```python
from build123d import *

# Parameters (mm, degrees)
F0_R         = 12.5
F1_DEPTH     = 12.5
F2_R         = 2.25
F3_DEPTH     = 25
F4_R         = 12.5
F5_DEPTH     = 7.5
F6_R         = 12.5
F7_DEPTH     = 7.5
F8_T4_DEPTH  = 24.3016555368
F8_S5_R      = 12.5
F8_T6_DEPTH  = 15
F8_T11_DEPTH = 24.3016555368
F8_S12_R     = 12.5
F8_T13_DEPTH = 14
F8_T17_DEPTH = 24.3016555368
F8_S18_R     = 12.5
F8_T19_DEPTH = 15
F8_T24_DEPTH = 24.3016555368
F8_S25_R     = 12.5
F8_T26_DEPTH = 15
F8_T30_DEPTH = 24.3016555368
F8_S31_R     = 12.5
F8_T32_DEPTH = 15
F8_T37_DEPTH = 24.3016555368
F8_S38_R     = 12.5
F8_T39_DEPTH = 15
F8_T44_DEPTH = 24.3016555368
F8_S45_R     = 12.5
F8_T46_DEPTH = 15
F9_T1_DEPTH  = 24.050587715
F9_T3_DEPTH  = 24.050587715
F9_T5_DEPTH  = 24.050587715
F9_T7_DEPTH  = 24.050587715
F9_T9_DEPTH  = 24.050587715
F9_T11_DEPTH = 24.050587715
F9_T13_DEPTH = 24.050587715
F10_R        = 2.5
F11_DEPTH    = 12


# Not quite as in the source:
# - a fillet or chamfer that OpenCascade refuses, or shapes differently, is made with other operations: its cross-section is extruded or revolved along the edge and cut away or added


with BuildPart() as f1:
    # F0 (on Top) → F1 (new body, symmetric)
    with BuildSketch(Plane.XY):
        Polygon((22.5, -5.1354781738), (22.5, 5.1354781738), (18.0435990556, 14.3892900865), (10.013442028, 20.7931266245), (0, 23.0786294236), (-10.013442028, 20.7931266245), (-18.0435990556, 14.3892900865), (-22.5, 5.1354781738), (-22.5, -5.1354781738), (-18.0435990556, -14.3892900865), (-10.013442028, -20.7931266245), (0, -23.0786294236), (10.013442028, -20.7931266245), (18.0435990556, -14.3892900865), align=None)
        Circle(F0_R, mode=Mode.SUBTRACT)
    extrude(amount=F1_DEPTH, both=True)

    # F2 (on face) → F3 (cut)
    with BuildSketch(Plane.XY.offset(12.5)):
        with Locations((9, 15.5884572681)):
            Circle(F2_R)
        with Locations((-18, 0)):
            Circle(F2_R)
        with Locations((9, -15.5884572681)):
            Circle(F2_R)
    extrude(amount=-F3_DEPTH, mode=Mode.SUBTRACT)

    # F4 (on face) → F5 (cut)
    with BuildSketch(Plane.XY.offset(12.5)):
        Polygon((14.9, -3.4008277684), (14.9, 3.4008277684), (11.9488722635, 9.5289076573), (6.6311238319, 13.7696705203), (0, 15.2831812628), (-6.6311238319, 13.7696705203), (-11.9488722635, 9.5289076573), (-14.9, 3.4008277684), (-14.9, -3.4008277684), (-11.9488722635, -9.5289076573), (-6.6311238319, -13.7696705203), (0, -15.2831812628), (6.6311238319, -13.7696705203), (11.9488722635, -9.5289076573), align=None)
        Circle(F4_R, mode=Mode.SUBTRACT)
    extrude(amount=-F5_DEPTH, mode=Mode.SUBTRACT)

    # F6 (on face) → F7 (join)
    with BuildSketch(Plane(origin=(0, 0, -12.5), x_dir=(1, 0, 0), z_dir=(0, 0, -1))):
        Polygon((14.35, -3.2752938575), (14.35, 3.2752938575), (11.5078065088, 9.1771694552), (6.3863508045, 13.2613940917), (0, 14.719036988), (-6.3863508045, 13.2613940917), (-11.5078065088, 9.1771694552), (-14.35, 3.2752938575), (-14.35, -3.2752938575), (-11.5078065088, -9.1771694552), (-6.3863508045, -13.2613940917), (0, -14.719036988), (6.3863508045, -13.2613940917), (11.5078065088, -9.1771694552), align=None)
        Circle(F6_R, mode=Mode.SUBTRACT)
    extrude(amount=F7_DEPTH)

    # F8: fillet of radius 3.5 on 7 edges, made by hand


with BuildPart() as f8_tool2:
    # F8_s3 → F8_t4 (new body)
    with BuildSketch(Plane(origin=(9.4998996874, 7.5759171977, 0), x_dir=(0, 0, 1), z_dir=(-0.7818314825, -0.6234898019, 0))):
        with BuildLine():
            ThreePointArc((5, 11.4), (6.0251262658, 13.8748737342), (8.5, 14.9))
            Line((8.5, 14.9), (5, 14.9))
            Line((5, 14.9), (5, 11.4))
        make_face()
    extrude(amount=F8_T4_DEPTH)

    # F8_s5 → F8_t6 (cut, symmetric)
    with BuildSketch(Plane.XY.offset(6.8)):
        Circle(F8_S5_R)
    extrude(amount=F8_T6_DEPTH, both=True, mode=Mode.SUBTRACT)

    split(bisect_by=Plane(origin=(-13.4244361317, 6.4648677129, 0), x_dir=(0, 0, 1), z_dir=(0.9009688679, -0.4338837391, 0)), keep=Keep.TOP)


with BuildPart() as f1_1:
    add(f1.part)

    # F8_t1: union F8_tool2
    add(f8_tool2.part)


with BuildPart() as f8_tool9:
    # F8_s10 → F8_t11 (new body)
    with BuildSketch(Plane.XZ.offset(-12.1508277684)):
        with BuildLine():
            ThreePointArc((-11.4, 5), (-13.8748737342, 6.0251262658), (-14.9, 8.5))
            Line((-14.9, 8.5), (-14.9, 5))
            Line((-14.9, 5), (-11.4, 5))
        make_face()
    extrude(amount=F8_T11_DEPTH)

    # F8_s12 → F8_t13 (cut, symmetric)
    with BuildSketch(Plane.XY.offset(6.8)):
        Circle(F8_S12_R)
    extrude(amount=F8_T13_DEPTH, both=True, mode=Mode.SUBTRACT)


with BuildPart() as f1_2:
    add(f1_1.part)

    # F8_t8: union F8_tool9
    add(f8_tool9.part)


with BuildPart() as f8_tool15:
    # F8_s16 → F8_t17 (new body)
    with BuildSketch(Plane(origin=(-9.4998996874, 7.5759171977, 0), x_dir=(0, 0, 1), z_dir=(0.7818314825, -0.6234898019, 0))):
        with BuildLine():
            ThreePointArc((5, 11.4), (6.0251262658, 13.8748737342), (8.5, 14.9))
            Line((8.5, 14.9), (5, 14.9))
            Line((5, 14.9), (5, 11.4))
        make_face()
    extrude(amount=F8_T17_DEPTH)

    # F8_s18 → F8_t19 (cut, symmetric)
    with BuildSketch(Plane.XY.offset(6.8)):
        Circle(F8_S18_R)
    extrude(amount=F8_T19_DEPTH, both=True, mode=Mode.SUBTRACT)

    split(bisect_by=Plane.YZ.offset(-14.9), keep=Keep.TOP)


with BuildPart() as f1_3:
    add(f1_2.part)

    # F8_t14: union F8_tool15
    add(f8_tool15.part)


with BuildPart() as f8_tool22:
    # F8_s23 → F8_t24 (new body)
    with BuildSketch(Plane(origin=(-11.8461811475, -2.7038135434, 0), x_dir=(0, 0, 1), z_dir=(0.9749279122, 0.222520934, 0))):
        with BuildLine():
            ThreePointArc((8.5, 14.9), (6.0251262658, 13.8748737342), (5, 11.4))
            Line((5, 11.4), (5, 14.9))
            Line((5, 14.9), (8.5, 14.9))
        make_face()
    extrude(amount=F8_T24_DEPTH)

    # F8_s25 → F8_t26 (cut, symmetric)
    with BuildSketch(Plane.XY.offset(6.8)):
        Circle(F8_S25_R)
    extrude(amount=F8_T26_DEPTH, both=True, mode=Mode.SUBTRACT)


with BuildPart() as f1_4:
    add(f1_3.part)

    # F8_t21: union F8_tool22
    add(f8_tool22.part)


with BuildPart() as f8_tool28:
    # F8_s29 → F8_t30 (new body)
    with BuildSketch(Plane(origin=(-5.2720465855, -10.9475175386, 0), x_dir=(0, 0, 1), z_dir=(0.4338837391, 0.9009688679, 0))):
        with BuildLine():
            ThreePointArc((5, 11.4), (6.0251262658, 13.8748737342), (8.5, 14.9))
            Line((8.5, 14.9), (5, 14.9))
            Line((5, 14.9), (5, 11.4))
        make_face()
    extrude(amount=F8_T30_DEPTH)

    # F8_s31 → F8_t32 (cut, symmetric)
    with BuildSketch(Plane.XY.offset(6.8)):
        Circle(F8_S31_R)
    extrude(amount=F8_T32_DEPTH, both=True, mode=Mode.SUBTRACT)

    split(bisect_by=Plane(origin=(9.2899980477, -11.6492890888, 0), x_dir=(0, 0, 1), z_dir=(-0.6234898019, 0.7818314825, 0)), keep=Keep.TOP)


with BuildPart() as f1_5:
    add(f1_4.part)

    # F8_t27: union F8_tool28
    add(f8_tool28.part)


with BuildPart() as f8_tool35:
    # F8_s36 → F8_t37 (new body)
    with BuildSketch(Plane(origin=(5.2720465855, -10.9475175386, 0), x_dir=(0, 0, 1), z_dir=(-0.4338837391, 0.9009688679, 0))):
        with BuildLine():
            ThreePointArc((5, 11.4), (6.0251262658, 13.8748737342), (8.5, 14.9))
            Line((8.5, 14.9), (5, 14.9))
            Line((5, 14.9), (5, 11.4))
        make_face()
    extrude(amount=F8_T37_DEPTH)

    # F8_s38 → F8_t39 (cut, symmetric)
    with BuildSketch(Plane.XY.offset(6.8)):
        Circle(F8_S38_R)
    extrude(amount=F8_T39_DEPTH, both=True, mode=Mode.SUBTRACT)

    split(bisect_by=Plane(origin=(9.2899980477, 11.6492890888, 0), x_dir=(0, 0, 1), z_dir=(-0.6234898019, -0.7818314825, 0)), keep=Keep.TOP)


with BuildPart() as f1_6:
    add(f1_5.part)

    # F8_t34: union F8_tool35
    add(f8_tool35.part)


with BuildPart() as f8_tool42:
    # F8_s43 → F8_t44 (new body)
    with BuildSketch(Plane(origin=(11.8461811475, -2.7038135434, 0), x_dir=(0, 0, 1), z_dir=(-0.9749279122, 0.222520934, 0))):
        with BuildLine():
            ThreePointArc((5, 11.4), (6.0251262658, 13.8748737342), (8.5, 14.9))
            Line((8.5, 14.9), (5, 14.9))
            Line((5, 14.9), (5, 11.4))
        make_face()
    extrude(amount=F8_T44_DEPTH)

    # F8_s45 → F8_t46 (cut, symmetric)
    with BuildSketch(Plane.XY.offset(6.8)):
        Circle(F8_S45_R)
    extrude(amount=F8_T46_DEPTH, both=True, mode=Mode.SUBTRACT)


with BuildPart() as f1_7:
    add(f1_6.part)

    # F8_t41: union F8_tool42
    add(f8_tool42.part)

    # F9: fillet of radius 3.5 on 7 edges, made by hand

    # F9_s2 → F9_t1 (cut)
    with BuildSketch(Plane(origin=(-5.2175794629, 10.834415393, 0), x_dir=(0, 0, 1), z_dir=(0.4338837391, -0.9009688679, 0))):
        with BuildLine():
            ThreePointArc((-16.5, -14.35), (-18.9748737342, -13.3248737342), (-20, -10.85))
            Line((-20, -10.85), (-20, -14.35))
            Line((-20, -14.35), (-16.5, -14.35))
        make_face()
    extrude(amount=F9_T1_DEPTH, mode=Mode.SUBTRACT)

    # F9_s4 → F9_t3 (cut)
    with BuildSketch(Plane(origin=(-11.7237946339, 2.6758796203, 0), x_dir=(0, 0, 1), z_dir=(0.9749279122, -0.222520934, 0))):
        with BuildLine():
            ThreePointArc((-16.5, -14.35), (-18.9748737342, -13.3248737342), (-20, -10.85))
            Line((-20, -10.85), (-20, -14.35))
            Line((-20, -14.35), (-16.5, -14.35))
        make_face()
    extrude(amount=F9_T3_DEPTH, mode=Mode.SUBTRACT)

    # F9_s6 → F9_t5 (cut)
    with BuildSketch(Plane(origin=(-9.4017533237, -7.4976480845, 0), x_dir=(0, 0, 1), z_dir=(0.7818314825, 0.6234898019, 0))):
        with BuildLine():
            ThreePointArc((-16.5, -14.35), (-18.9748737342, -13.3248737342), (-20, -10.85))
            Line((-20, -10.85), (-20, -14.35))
            Line((-20, -14.35), (-16.5, -14.35))
        make_face()
    extrude(amount=F9_T5_DEPTH, mode=Mode.SUBTRACT)

    # F9_s8 → F9_t7 (cut)
    with BuildSketch(Plane.XZ.offset(-12.0252938575)):
        with BuildLine():
            ThreePointArc((-14.35, -16.5), (-13.3248737342, -18.9748737342), (-10.85, -20))
            Line((-10.85, -20), (-14.35, -20))
            Line((-14.35, -20), (-14.35, -16.5))
        make_face()
    extrude(amount=F9_T7_DEPTH, mode=Mode.SUBTRACT)

    # F9_s10 → F9_t9 (cut)
    with BuildSketch(Plane(origin=(9.4017533237, -7.4976480845, 0), x_dir=(0, 0, 1), z_dir=(-0.7818314825, 0.6234898019, 0))):
        with BuildLine():
            ThreePointArc((-16.5, -14.35), (-18.9748737342, -13.3248737342), (-20, -10.85))
            Line((-20, -10.85), (-20, -14.35))
            Line((-20, -14.35), (-16.5, -14.35))
        make_face()
    extrude(amount=F9_T9_DEPTH, mode=Mode.SUBTRACT)

    # F9_s12 → F9_t11 (cut)
    with BuildSketch(Plane(origin=(11.7237946339, 2.6758796203, 0), x_dir=(0, 0, 1), z_dir=(-0.9749279122, -0.222520934, 0))):
        with BuildLine():
            ThreePointArc((-16.5, -14.35), (-18.9748737342, -13.3248737342), (-20, -10.85))
            Line((-20, -10.85), (-20, -14.35))
            Line((-20, -14.35), (-16.5, -14.35))
        make_face()
    extrude(amount=F9_T11_DEPTH, mode=Mode.SUBTRACT)

    # F9_s14 → F9_t13 (cut)
    with BuildSketch(Plane(origin=(5.2175794629, 10.834415393, 0), x_dir=(0, 0, 1), z_dir=(-0.4338837391, -0.9009688679, 0))):
        with BuildLine():
            ThreePointArc((-16.5, -14.35), (-18.9748737342, -13.3248737342), (-20, -10.85))
            Line((-20, -10.85), (-20, -14.35))
            Line((-20, -14.35), (-16.5, -14.35))
        make_face()
    extrude(amount=F9_T13_DEPTH, mode=Mode.SUBTRACT)

    # F10 (on face) → F11 (cut)
    with BuildSketch(Plane.YZ.offset(22.5)):
        Circle(F10_R)
    extrude(amount=-F11_DEPTH, mode=Mode.SUBTRACT)


solid = f1_7.part
```
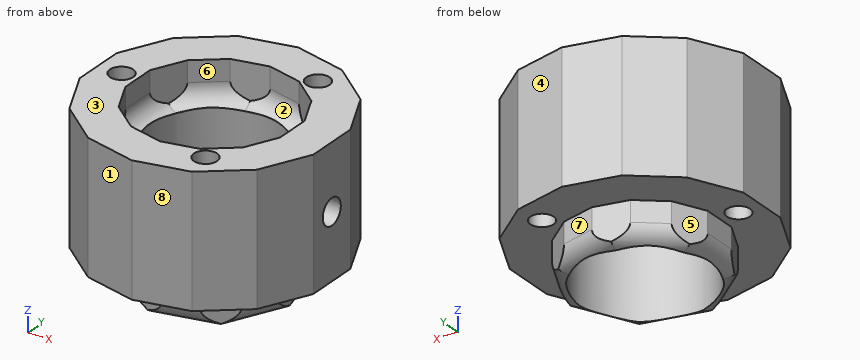
Build history of the part. All positions in model axes, mm. Face numbers are marked on the shaded views. A direction names the side the tool comes from. Round coordinates to 2 decimals unless told otherwise and drop trailing zeros. Order: outer loops, then holes, each group sorted by start corner. A loop starts at its lowest first (then second) coordinate and runs counter-clockwise, first axis right, second up. Notation, with made-up numbers: (41.5, -12) - (67.5, -12) arc R25 ccw to (67.5, 15) - close; hole circle Ø8 at (66, 1). An arc over 180 degrees is marked (long way). Use a Markdown table: item, result.
1) Tool access for the marked faces 4, 5, 6, 7 and 8: list every direction of +Z, -Z, +X, -X, +Y, -Y with a clear straight run to the whole face (end or side of a thin tool).
Recorded:
| item | result |
|---|---|
| face 4 | +Z, -Z, +X, +Y |
| face 5 | -Z, -X, +Y |
| face 6 | +Z |
| face 7 | -Z, +X, +Y |
| face 8 | +Z, -Z, +X, -Y |
2) Saw through at C-C on y = 19.5. Write the cut outline in (x, z).
Recorded:
| item | result |
|---|---|
| outline | (-11.63, -12.5) - (11.63, -12.5) - (11.63, 12.5) - (-11.63, 12.5) - close |
3) Pull direction Y, two halves, no side cores. Call the marked faces 1, 2 and 3: pulls with the +Y half, pulls with the -Y half, needs draft (parallel to the pull), parting line crosses it, or undercut.
Recorded:
| item | result |
|---|---|
| face 1 | pulls with the -Y half |
| face 2 | undercut |
| face 3 | needs draft |
4) Saw through at A-A on z = -1.5. Write the cut outline in (x, y), and give its area (3 significant figures).
Recorded:
| item | result |
|---|---|
| outline | (-22.5, -5.14) - (-18.04, -14.39) - (-10.01, -20.79) - (0, -23.08) - (10.01, -20.79) - (18.04, -14.39) - (22.5, -5.14) - (22.5, -2) - (12.34, -2) arc R12.5 cw (long way) to (12.34, 2) - (22.5, 2) - (22.5, 5.14) - (18.04, 14.39) - (10.01, 20.79) - (0, 23.08) - (-10.01, 20.79) - (-18.04, 14.39) - (-22.5, 5.14) - close; hole circle Ø4.5 at (-18, 0); hole circle Ø4.5 at (9, -15.59); hole circle Ø4.5 at (9, 15.59) |
| area | 1,040 mm² |
5) Saw through at B-B on z = -6. Write the cut outline in (x, y).
Recorded:
| item | result |
|---|---|
| outline | (-22.5, -5.14) - (-18.04, -14.39) - (-10.01, -20.79) - (0, -23.08) - (10.01, -20.79) - (18.04, -14.39) - (22.5, -5.14) - (22.5, 5.14) - (18.04, 14.39) - (10.01, 20.79) - (0, 23.08) - (-10.01, 20.79) - (-18.04, 14.39) - (-22.5, 5.14) - close; hole circle Ø4.5 at (-18, 0); hole circle Ø25 at (0, 0); hole circle Ø4.5 at (9, -15.59); hole circle Ø4.5 at (9, 15.59) |
6) Wall check: L1, parallel to Y at x = 0, z = -3.75; L2, parallel to Y at x = 9, z = -7; L3, parallel to Y at x = 10, z = 2.5. Give the ranges that are in metal, low to high.
Recorded:
| item | result |
|---|---|
| L1 | y = -23.08 to -12.5, 12.5 to 23.08 |
| L2 | y = -21.02 to -17.84, -13.34 to -8.67, 8.67 to 13.34, 17.84 to 21.02 |
| L3 | y = -20.8 to -17.6, -13.57 to -7.5, 7.5 to 13.57, 17.6 to 20.8 |
7) Flat gauge pins, fed straight in: pin 1 Ø3 at (y, z) = (0, 0) entering from +X; pin 2 Ø12 at (x, z) = (1.5, 6) entering from +Y; pin 3 Ø10 at (x, z) = (6, -10) entering from +Y; pin 4 Ø2.5 at (x, y) = (9, 15.59) entering from +Z. Where does each tip first touch, or does it go through?
Recorded:
| item | result |
|---|---|
| pin 1 | stops at x = -12.41 |
| pin 2 | stops at y = 23.08 |
| pin 3 | stops at y = 22.85 |
| pin 4 | passes through |
